Verification items for the finished model (mm, model axes). Coordinates: 2 decimals unless noted, no trailing zeros. Write each loop counter-clockwise with the first axis right and the second up, starting at its lowest first coordinate (ties: lowest second). Pieces come first, ordered by that corner, then holes. Notation, with made-up numbers: (4.25, -33.75) - (54.25, -33.75) arc R24 ccw to (54.25, 1.25) - close; hole circle Ø8 at (6.5, 4.5). An arc over 180 degrees is marked (long way). Use one line per item in the form item = value. Start each with the question number.
(1) Mould release check, pull along Y, two halves, no side actions. Record for faces 1 (the cylindrical face through (8.375, 1.293, 2.535)), 2 (the flat face through (38.1, 1, 2)), 3 (the flat face through (19, 0, 2)): released by +Y, released by -Y, zero draft, split by the parting line, or undercut.
(2) Material ranges on line 1 (Y direction, x = 29.21, z = 3.1); line 2 (Y direction, x = 34, z = 0.9), recorded low to high. Write a range as [from, to].
(3) Sectioned sample at B-B (z = 0.55). Count the separate pieces of the cut face and the enclosed holes in it, and give its area (3 significant figures).
(4) Sectioned sample at A-A (x = 31.75). Record the cut outline in (y, z).
(5) Gauge pin test, flat ends, axial feed: pin 1 Ø1.2 at (x, y) = (11.43, 1.27) entering from +Z; pin 2 Ø0.9 at (x, y) = (13.97, 1.27) entering from +Z. Record the tip position at first contact, or that the pin passes through.
from build123d import *

# Parameters (mm, degrees)
SKETCH1_W           = 38.1
SKETCH1_H           = 2.54
BOSS_EXTRUDE1_DEPTH = 5
SKETCH2_R           = 0.515143842
CUT_EXTRUDE1_DEPTH  = 39.510538817


with BuildPart() as part:
    # Sketch1 → Boss-Extrude1 (new body)
    with BuildSketch(Plane.XY):
        with Locations((19.05, 1.27)):
            Rectangle(SKETCH1_W, SKETCH1_H)
    extrude(amount=BOSS_EXTRUDE1_DEPTH)

    # Sketch2 → Cut-Extrude1 (cut, through all)
    with BuildSketch(Plane.XY.offset(5)):
        with Locations((1.27, 1.27)):
            Circle(SKETCH2_R)
        with Locations((3.81, 1.27)):
            Circle(SKETCH2_R)
        with Locations((6.35, 1.27)):
            Circle(SKETCH2_R)
        with Locations((8.89, 1.27)):
            Circle(SKETCH2_R)
        with Locations((11.43, 1.27)):
            Circle(SKETCH2_R)
        with Locations((13.97, 1.27)):
            Circle(SKETCH2_R)
        with Locations((16.51, 1.27)):
            Circle(SKETCH2_R)
        with Locations((19.05, 1.27)):
            Circle(SKETCH2_R)
        with Locations((21.59, 1.27)):
            Circle(SKETCH2_R)
        with Locations((24.13, 1.27)):
            Circle(SKETCH2_R)
        with Locations((26.67, 1.27)):
            Circle(SKETCH2_R)
        with Locations((29.21, 1.27)):
            Circle(SKETCH2_R)
        with Locations((31.75, 1.27)):
            Circle(SKETCH2_R)
        with Locations((34.29, 1.27)):
            Circle(SKETCH2_R)
        with Locations((36.83, 1.27)):
            Circle(SKETCH2_R)
    extrude(amount=-CUT_EXTRUDE1_DEPTH, mode=Mode.SUBTRACT)


solid = part.part
Answers below:
q1.face_1 = undercut
q1.face_2 = zero draft
q1.face_3 = released by -Y
q2.line_1 = [0, 0.75], [1.79, 2.54]
q2.line_2 = [0, 0.84], [1.7, 2.54]
q3.separate_pieces = 1
q3.enclosed_holes = 15
q3.area = 84.3 mm2
q4.outline = (0, 0) - (0.75, 0) - (0.75, 5) - (0, 5) - close; (1.79, 0) - (2.54, 0) - (2.54, 5) - (1.79, 5) - close
q5.pin_1 = 5
q5.pin_2 = through
